from build123d import *

# Parameters (mm, degrees)
SKETCH_1_W          = 96
SKETCH_1_H          = 96
EXTRUDE_1_DEPTH     = 10
SKETCH_2_R          = 3.5
CUT_EXTRUDE_1_DEPTH = 10
SKETCH_3_R          = 3.5
CUT_EXTRUDE_2_DEPTH = 10
CUT_EXTRUDE_3_DEPTH = 10
SKETCH_5_R          = 3.5
CUT_EXTRUDE_4_DEPTH = 10


with BuildPart() as part:
    # 草图1 → 凸台-拉伸1 (new body)
    with BuildSketch(Plane(origin=(0, 0, 0), x_dir=(1, 0, 0), z_dir=(0, 1, 0))):
        Rectangle(SKETCH_1_W, SKETCH_1_H)
    extrude(amount=EXTRUDE_1_DEPTH)

    # 草图2 → 切除-拉伸1 (cut)
    with BuildSketch(Plane.XY.offset(48)):
        with Locations((0, 5)):
            Circle(SKETCH_2_R)
    extrude(amount=-CUT_EXTRUDE_1_DEPTH, mode=Mode.SUBTRACT)

    # 草图3 → 切除-拉伸2 (cut)
    with BuildSketch(Plane(origin=(48, 0, 0), x_dir=(0, 0, -1), z_dir=(1, 0, 0))):
        with Locations((0, 5)):
            Circle(SKETCH_3_R)
    extrude(amount=-CUT_EXTRUDE_2_DEPTH, mode=Mode.SUBTRACT)

    # 草图4 → 切除-拉伸3 (cut)
    with BuildSketch(Plane(origin=(0, 0, -48), x_dir=(-1, 0, 0), z_dir=(0, 0, -1))):
        with BuildLine():
            ThreePointArc((3.481164431, 5.362621295), (0, 8.5), (-3.481164431, 5.362621295))
            Line((-3.481164431, 5.362621295), (0, 5))
            Line((0, 5), (3.481164431, 5.362621295))
        make_face()
        with BuildLine():
            Line((0, 5), (-3.481164431, 5.362621295))
            ThreePointArc((-3.481164431, 5.362621295), (-3.5, 5), (-3.481164431, 4.637378705))
            Line((-3.481164431, 4.637378705), (0, 5))
        make_face()
        with BuildLine():
            Line((3.481164431, 5.362621295), (0, 5))
            Line((0, 5), (3.481164431, 4.637378705))
            ThreePointArc((3.481164431, 4.637378705), (3.495287936, 4.818444924), (3.5, 5))
            ThreePointArc((3.5, 5), (3.495287936, 5.181555076), (3.481164431, 5.362621295))
        make_face()
        with BuildLine():
            Line((3.481164431, 4.637378705), (0, 5))
            Line((0, 5), (-3.481164431, 4.637378705))
            ThreePointArc((-3.481164431, 4.637378705), (0, 1.5), (3.481164431, 4.637378705))
        make_face()
    extrude(amount=-CUT_EXTRUDE_3_DEPTH, mode=Mode.SUBTRACT)

    # 草图5 → 切除-拉伸4 (cut)
    with BuildSketch(Plane.ZY.offset(48)):
        with Locations((0, 5)):
            Circle(SKETCH_5_R)
    extrude(amount=-CUT_EXTRUDE_4_DEPTH, mode=Mode.SUBTRACT)


solid = part.part
Input: part model. Units: mm. Frame: model coordinates. A direction names the side the tool comes from. Give positions to 0.01 mm unless a question says otherwise; leave off trailing zeros. Order: outer loops, then holes, each group sorted by start corner. A loop starts at its lowest first (then second) coordinate and runs counter-clockwise, first axis right, second up.
Q1. Section A-A on z = 0. Output: boundary loops of the cut face in (x, y).
Checked values:
outline: (-48, 0) - (48, 0) - (48, 1.5) - (38, 1.5) - (38, 8.5) - (48, 8.5) - (48, 10) - (-48, 10) - (-48, 8.5) - (-38, 8.5) - (-38, 1.5) - (-48, 1.5) - close
Q2. Contact query for flat-ended pins moving along their axis: pin 1 Ø2 at (x, y) = (0, 3.5) entering from -Z; pin 2 Ø5.5 at (y, z) = (5, 0) entering from +X; pin 3 Ø3.5 at (x, y) = (0.5, 6.5) entering from +Z. Output: stop coordinate, or through.
Checked values:
pin 1: stops at z = -38
pin 2: stops at x = 38
pin 3: stops at z = 38
Q3. Ray query, probe 1 along Y at (x, z) = (41.75, 0); probe 2 along Z at (x, y) = (44, 2.5); probe 3 along Z at (x, y) = (-39, 7.25). Return the intervals inside material, ascending.
Checked values:
probe 1: y = 0 to 1.5, 8.5 to 10
probe 2: z = -48 to -2.45, 2.45 to 48
probe 3: z = -48 to -2.68, 2.68 to 48
Q4. Draft query along Y for faces 6 (the flat face through (0, 5, -38)), 7 (the flat face through (-1, 10, -1)), 8 (the flat face through (-48, 0.5, 0.7)). Return one class per face: +Y half, -Y half, draft (parallel to the pull), parting line (faces both ways), or undercut.
Checked values:
face 6: undercut
face 7: +Y half
face 8: draft
Q5. Set-up query: faces 1 (the flat face through (0, 5, 38)), 2 (the flat face through (38, 5, 0)), 3 (the flat face through (48, 0.5, 0.7)), 4 (the flat face through (-0.7, 0.5, -48)), 5 (the flat face through (-38, 5, 0)). Return all of +Z, -Z, +X, -X, +Y, -Y with unobstructed straight access to the full face (end or side cutting, diameter ignored); none if empty.
Checked values:
face 1: +Z
face 2: +X
face 3: +Z, -Z, +X, +Y, -Y
face 4: -Z, +X, -X, +Y, -Y
face 5: -X
